```python
from build123d import *

# Parameters (mm, degrees)
SKETCH1_W                    = 20
SKETCH1_H                    = 5
SKETCH1_H_2                  = 12
BOSS_EXTRUDE1_DEPTH          = 5
SKETCH2_W                    = 20
SKETCH2_H                    = 15
BOSS_EXTRUDE2_DEPTH          = 5
F_5_0_5_DIAMETER_HOLE1_D     = 5
F_5_0_5_DIAMETER_HOLE1_DEPTH = 5
F_4_5_M4_HEAT_SET_D          = 4.8
F_4_5_M4_HEAT_SET_DEPTH      = 5
FILLET1_R                    = 3


with BuildPart() as part:
    # Sketch1 → Boss-Extrude1 (new body)
    with BuildSketch(Plane(origin=(0, 0, 0), x_dir=(1, 0, 0), z_dir=(0, 1, 0))):
        with Locations((0, 8.5)):
            Rectangle(SKETCH1_W, SKETCH1_H)
        Rectangle(SKETCH1_W, SKETCH1_H_2)
        with Locations((0, -8.5)):
            Rectangle(SKETCH1_W, SKETCH1_H)
    extrude(amount=BOSS_EXTRUDE1_DEPTH)

    # Sketch2 → Boss-Extrude2 (add)
    with BuildSketch(Plane.XY.offset(11)):
        with Locations((0, 12.5)):
            Rectangle(SKETCH2_W, SKETCH2_H)
    extrude(amount=-BOSS_EXTRUDE2_DEPTH)

    # Ø5.0 (5) Diameter Hole1
    with Locations(Plane(origin=(0, 5, 0), x_dir=(1, 0, 0), z_dir=(0, 1, 0))):
        with Locations((0, 0)):
            Hole(F_5_0_5_DIAMETER_HOLE1_D / 2, depth=F_5_0_5_DIAMETER_HOLE1_DEPTH)

    # Ø4.5 M4 heat set
    with Locations(Plane(origin=(0, 0, 6), x_dir=(1, 0, 0), z_dir=(0, 0, -1))):
        with Locations((0, -12.5)):
            Hole(F_4_5_M4_HEAT_SET_D / 2, depth=F_4_5_M4_HEAT_SET_DEPTH)

    # Fillet1
    fillet1_edges = [part.edges().sort_by_distance(p)[0] for p in [
        (0, 5, 6),
    ]]
    fillet(fillet1_edges, radius=FILLET1_R)


solid = part.part
```
Verification items for the finished model (mm, model axes). A direction names the side the tool comes from. Give positions to 0.01 mm unless a question says otherwise; leave off trailing zeros. Order: outer loops, then holes, each group sorted by start corner. A loop starts at its lowest first (then second) coordinate and runs counter-clockwise, first axis right, second up. Notation, with made-up numbers: M 14.25,71 L 20.25,71 A23 ccw 20.25,109 Z; hole C -1.75,-8.5 d1. An arc over 180 degrees is marked long. Return JSON: item names as keys, results as strings. Group by question number.
1) Section check C-C on x = 0. Record the cut outline in (y, z), and give its area (3 significant figures).
2) Scan lines: line 1 (Z direction, x = 0, y = 3.2); line 2 (X direction, y = 12.5, z = 7.6); line 3 (Y direction, x = 0, z = 7.85). Record each from-to range of solid material in increasing order.
3) Section check D-D on y = 3.5. Record the cut outline in (x, z).
4) Section check A-A on z = 0. Record the cut outline in (x, y), and give its area (3 significant figures).
5) Mould release check, pull along X, two halves, no side actions. Record for faces 3 (the face through (0.14, 5.86, 5.1)), 4 (the face through (0.54, 2.46, 2.44)), 5 (the face through (-10, 5, 5)), 6 (the face through (10, 5, 5)): pulls with the +X half, pulls with the -X half, needs draft (parallel to the pull), parting line crosses it, or undercut.
6) Go/stop test with flat-tipped pins: pin 1 Ø6 at (x, y) = (-2.5, 13) entering from -Z; pin 2 Ø1.5 at (x, z) = (-6.5, 2.5) entering from +Y; pin 3 Ø12 at (x, z) = (4, 1.5) entering from +Y; pin 4 Ø3 at (x, y) = (0, 12.5) entering from -Z. Record where each tip stops, or that it passes through.
7) Section check B-B on y = 12.5. Record the cut outline in (x, z), and give its area (3 significant figures).
8) Access from +Z, -Z, +X, -X, +Y, -Y to the whole of each face (thin tool, end or side, straight path). Record for faces 1 (the face through (0, 20, 9)), 2 (the face through (-0.1, 15.4, 6)).
Answer block:
{
 "1": {"outline": "M 0,-11 L 5,-11 L 5,-2.5 L 0,-2.5 Z; M 0,2.5 L 5,2.5 L 5,3 A3 cw 8,6 L 10.1,6 L 10.1,11 L 0,11 Z; M 14.9,6 L 20,6 L 20,11 L 14.9,11 Z", "area": "138 mm^2"},
 "2": {"line 1": "z = -11 to -2.5, 2.5 to 11", "line 2": "x = -10 to -2.4, 2.4 to 10", "line 3": "y = 0 to 10.1, 14.9 to 20"},
 "3": {"outline": "M -10,-11 L 10,-11 L 10,11 L -10,11 Z; hole C 0,0 d5"},
 "4": {"outline": "M -10,0 L -2.5,0 L -2.5,5 L -10,5 Z; M 2.5,0 L 10,0 L 10,5 L 2.5,5 Z", "area": "75.0 mm^2"},
 "5": {"face 3": "needs draft", "face 4": "undercut", "face 5": "pulls with the -X half", "face 6": "pulls with the +X half"},
 "6": {"pin 1": "stops at z = 6", "pin 2": "stops at y = 5.01", "pin 3": "stops at y = 20", "pin 4": "passes through"},
 "7": {"outline": "M -10,6 L -2.4,6 L -2.4,11 L -10,11 Z; M 2.4,6 L 10,6 L 10,11 L 2.4,11 Z", "area": "76.0 mm^2"},
 "8": {"face 1": "+Z, -Z, +X, -X, +Y", "face 2": "-Z, +X, -X, +Y"}
}
